Check sheet for the modelled part. Datum: model origin and axes. Units: mm. Face numbers are marked on the shaded views. A direction names the side the tool comes from. Round coordinates to 2 decimals unless told otherwise and drop trailing zeros. Order: outer loops, then holes, each group sorted by start corner. A loop starts at its lowest first (then second) coordinate and runs counter-clockwise, first axis right, second up. Notation, with made-up numbers: (-12.5, 69) -> (6.5, 69) arc R27 ccw to (6.5, 100) -> close; hole circle Ø10 at (34, -9.5). An arc over 180 degrees is marked (long way). Answer in a Markdown table with one row per item.
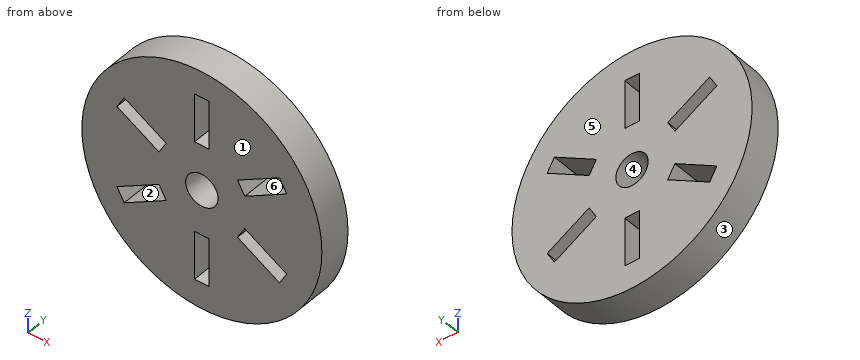
```python
from build123d import *

# Parameters (mm, degrees)
F0_R     = 47.049259
F0_W     = 5.6896
F0_H     = 18.983845
F0_R_2   = 6.35
F1_DEPTH = 12.7


with BuildPart() as f1:
    # F0 (on Front) → F1 (new body)
    with BuildSketch(Plane.XZ):
        Circle(F0_R)
        Polygon((-33.26515, -15.920751), (-16.824658, -6.428829), (-13.979858, -11.356167), (-30.42035, -20.848089), align=None, mode=Mode.SUBTRACT)
        with Locations((0, -27.276919)):
            Rectangle(F0_W, F0_H, mode=Mode.SUBTRACT)
        Polygon((30.42035, -20.848089), (13.979858, -11.356167), (16.824658, -6.428829), (33.26515, -15.920751), align=None, mode=Mode.SUBTRACT)
        Polygon((-30.42035, 20.848089), (-13.979858, 11.356167), (-16.824658, 6.428829), (-33.26515, 15.920751), align=None, mode=Mode.SUBTRACT)
        Circle(F0_R_2, mode=Mode.SUBTRACT)
        Polygon((33.26515, 15.920751), (16.824658, 6.428829), (13.979858, 11.356167), (30.42035, 20.848089), align=None, mode=Mode.SUBTRACT)
        with Locations((0, 27.276919)):
            Rectangle(F0_W, F0_H, mode=Mode.SUBTRACT)
    extrude(amount=F1_DEPTH)


solid = f1.part
```
(1) Section check A-A on z = 0. Record the boundary of the cut face in (x, y).
Solutions:
| item | result |
|---|---|
| outline | (-47.05, -12.7) -> (-6.35, -12.7) -> (-6.35, 0) -> (-47.05, 0) -> close; (6.35, -12.7) -> (47.05, -12.7) -> (47.05, 0) -> (6.35, 0) -> close |
(2) Section check C-C on y = -7.25. Record the boundary of the cut face in (x, z) (3 decimals), plus the area to 3 significant figures.
Solutions:
| item | result |
|---|---|
| outline | circle Ø94.099 at (0, 0); hole (-33.265, -15.921) -> (-30.42, -20.848) -> (-13.98, -11.356) -> (-16.825, -6.429) -> close; hole (-33.265, 15.921) -> (-16.825, 6.429) -> (-13.98, 11.356) -> (-30.42, 20.848) -> close; hole circle Ø12.7 at (0, 0); hole (-2.845, -36.769) -> (2.845, -36.769) -> (2.845, -17.785) -> (-2.845, -17.785) -> close; hole (-2.845, 17.785) -> (2.845, 17.785) -> (2.845, 36.769) -> (-2.845, 36.769) -> close; hole (13.98, -11.356) -> (30.42, -20.848) -> (33.265, -15.921) -> (16.825, -6.429) -> close; hole (13.98, 11.356) -> (16.825, 6.429) -> (33.265, 15.921) -> (30.42, 20.848) -> close |
| area | 6,180 mm^2 |
(3) Scan lines: probe 1 along Z at (x, y) = (0, -5.75) (3 decimals); probe 2 along Z at (x, y) = (21.5, -0.75); probe 3 along Z at (x, y) = (-29.5, -7.5). Record each from-to range of solid material in increasing order. Write a range as from..to.
Solutions:
| item | result |
|---|---|
| probe 1 | -47.049..-36.769, -17.785..-6.35, 6.35..17.785, 36.769..47.049 |
| probe 2 | -41.85..-15.7, -9.13..9.13, 15.7..41.85 |
| probe 3 | -36.65..-20.32, -13.75..13.75, 20.32..36.65 |
(4) Draft check along X on the marked faces 3, 4, 5 and 6. Enter one of: pulls with the +X half, pulls with the -X half, needs draft (parallel to the pull), parting line crosses it, or undercut.
Solutions:
| item | result |
|---|---|
| face 3 | parting line crosses it |
| face 4 | undercut |
| face 5 | needs draft |
| face 6 | undercut |
(5) Tool access check on the marked faces 1 and 2. Record the directions out of +Z, -Z, +X, -X, +Y, -Y that give a thin tool (end or side, any length) a straight path to the whole face; none if there is none.
Solutions:
| item | result |
|---|---|
| face 1 | +Z, -Z, +X, -X, -Y |
| face 2 | +Y, -Y |
(6) Depth check by flat-ended pin: pin 1 Ø6.5 at (y, z) = (-8, -28.5) entering from -X; pin 2 Ø4.5 at (x, y) = (-1.5, -6) entering from -Z; pin 3 Ø1 at (y, z) = (-10, 27) entering from +X. Enter the tip coordinate at first touch or a pass-through.
Solutions:
| item | result |
|---|---|
| pin 1 | x = -39.7 |
| pin 2 | z = -47.05 |
| pin 3 | x = 38.88 |
(7) Section check D-D on z = 14.5. Record the boundary of the cut face in (x, y).
Solutions:
| item | result |
|---|---|
| outline | (-44.76, -12.7) -> (-30.8, -12.7) -> (-30.8, 0) -> (-44.76, 0) -> close; (-19.43, -12.7) -> (19.43, -12.7) -> (19.43, 0) -> (-19.43, 0) -> close; (30.8, -12.7) -> (44.76, -12.7) -> (44.76, 0) -> (30.8, 0) -> close |
(8) Section check B-B on x = 0. Record the boundary of the cut face in (y, z) (3 decimals).
Solutions:
| item | result |
|---|---|
| outline | (-12.7, -47.049) -> (0, -47.049) -> (0, -36.769) -> (-12.7, -36.769) -> close; (-12.7, -17.785) -> (0, -17.785) -> (0, -6.35) -> (-12.7, -6.35) -> close; (-12.7, 6.35) -> (0, 6.35) -> (0, 17.785) -> (-12.7, 17.785) -> close; (-12.7, 36.769) -> (0, 36.769) -> (0, 47.049) -> (-12.7, 47.049) -> close |
